Here's how the part is built. I have some questions about the finished solid (model axes, mm). Coordinates: 2 decimals unless noted, no trailing zeros. Loops run counter-clockwise (first coordinate to the right, second up) from the corner with the lowest first, then second, coordinate; pieces in that order, holes last. Notation, with made-up numbers: (5, 72) -> (49, 72) arc R26 ccw to (49, 104) -> close; hole circle Ø4 at (-34.5, 39). An arc over 180 degrees is marked (long way). Answer as a JSON object with one key per item and string values. Group by question number.
Q1. I need wall thicknesses on line 1 (Z direction, x = 0, y = -247); line 2 (Z direction, x = 2, y = -293.5); line 3 (Y direction, x = -1, z = -12.5). Which ranges of each line are inside material? Lowest first, please.
Q2. I want a section at A-A on y = -392. Write out the boundary of the cut face in (x, z), then the cut area to 3 significant figures.
Q3. I'm going to push flat-ended pins straight in: pin 1 (5.5 mm diameter, centred on x = -1, z = 13.5, fed in from -Y); pin 2 (3.5 mm diameter, centred on x = 1, z = -15, fed in from -Y). Where does each tip first touch, or does it pass through?
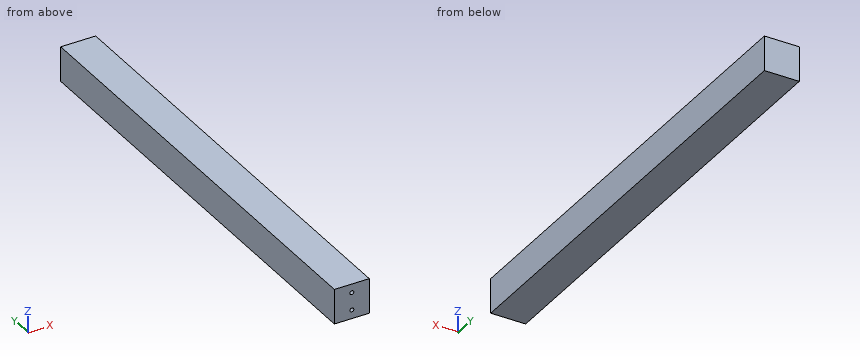
```python
from build123d import *

# Parameters (mm, degrees)
F0_W     = 60
F0_H     = 60
F1_DEPTH = 796.2
F2_W     = 60
F2_H     = 60
F3_DEPTH = 6
F4_R     = 3.4
F5_DEPTH = 796.201
F6_W     = 60
F6_H     = 60
F7_DEPTH = 6


with BuildPart() as f1:
    # F0 (on Front) → F1 (new body)
    with BuildSketch(Plane.XZ):
        Rectangle(F0_W, F0_H)
    extrude(amount=F1_DEPTH)

    # F2 (on face) → F3 (join)
    with BuildSketch(Plane.XZ.offset(796.2)):
        Rectangle(F2_W, F2_H)
    extrude(amount=-F3_DEPTH)

    # F4 (on face) → F5 (cut, through all)
    with BuildSketch(Plane.XZ.offset(796.2)):
        with Locations((0, 15)):
            Circle(F4_R)
        with Locations((0, -15)):
            Circle(F4_R)
    extrude(amount=-F5_DEPTH, mode=Mode.SUBTRACT)

    # F6 (on face) → F7 (join)
    with BuildSketch(Plane(origin=(0, 0, 0), x_dir=(-1, 0, 0), z_dir=(0, 1, 0))):
        Rectangle(F6_W, F6_H)
    extrude(amount=-F7_DEPTH)


solid = f1.part
```
Result set:
{
 "1": {"line 1": "z = -30 to -18.4, -11.6 to 11.6, 18.4 to 30", "line 2": "z = -30 to -17.75, -12.25 to 12.25, 17.75 to 30", "line 3": "y = -6 to 0"},
 "2": {"outline": "(-30, -30) -> (30, -30) -> (30, 30) -> (-30, 30) -> close; hole circle Ø6.8 at (0, -15); hole circle Ø6.8 at (0, 15)", "area": "3,530 mm²"},
 "3": {"pin 1": "stops at y = -796.2", "pin 2": "stops at y = -6"}
}
